For this review, take the finished solid that the model builds, in its own axes (mm). A direction names the side the tool comes from. Give positions to 0.01 mm unless a question says otherwise; leave off trailing zeros. Order: outer loops, then holes, each group sorted by start corner. A loop starts at its lowest first (then second) coordinate and runs counter-clockwise, first axis right, second up.
from build123d import *

# Parameters (mm, degrees)
SKETCH1_R           = 6.35
SKETCH1_R_2         = 7.62
BOSS_EXTRUDE1_DEPTH = 25.4
FILLET3_R           = 12.7


with BuildPart() as part:
    # Sketch1 → Boss-Extrude1 (new body)
    with BuildSketch(Plane.XY):
        Polygon((-106.967651581, 12.7), (103.301477372, 19.05), (125.298522628, 19.05), (136.297045256, 0), (125.298522628, -19.05), (103.301477372, -19.05), (-106.967651581, -12.7), (-121.632348419, -12.7), (-128.964696837, 0), (-121.632348419, 12.7), align=None)
        with Locations((-114.3, 0)):
            Circle(SKETCH1_R, mode=Mode.SUBTRACT)
        with Locations((114.3, 0)):
            Circle(SKETCH1_R_2, mode=Mode.SUBTRACT)
    extrude(amount=BOSS_EXTRUDE1_DEPTH)

    # Fillet3
    fillet3_edges = [part.edges().sort_by_distance(p)[0] for p in [
        (-128.964696837, 0, 12.7),
        (-121.632348419, 12.7, 12.7),
        (125.298522628, -19.05, 12.7),
        (136.297045256, 0, 12.7),
        (125.298522628, 19.05, 12.7),
        (-121.632348419, -12.7, 12.7),
    ]]
    fillet(fillet3_edges, radius=FILLET3_R - 0.0001)  # a hair under: the kernel refuses the full size


solid = part.part
1) To check wall thickness, follow line 1 (Y direction, x = 114.3, z = 13); line 2 (X direction, y = 1, z = 4.5); line 3 (Y direction, x = -114.3, z = 17.75). State the ranges of each line that lie inside material, in increasing order.
Answer sheet:
line 1: y = -19.05 to -7.62, 7.62 to 19.05
line 2: x = -126.96 to -120.57, -108.03 to 106.75, 121.85 to 134.29
line 3: y = -12.7 to -6.35, 6.35 to 12.7
2) Draft analysis for pull direction Y (two halves, no side actions). For faces 1 (the face through (124.4, -17.3, 12.9)), 2 (the face through (106.687, 0.335, 12.522)), 3 (the face through (134.332, 0.093, 12.878)), state which applies: +Y half, -Y half, draft (parallel to the pull), parting line (faces both ways), or undercut.
Answer sheet:
face 1: -Y half
face 2: undercut
face 3: parting line
3) Tool access review of faces 4 (the face through (-127, 0, 13)), 5 (the face through (-111, 12.7, 13)), 6 (the face through (-111, -12.7, 13)): name each direction out of +Z, -Z, +X, -X, +Y, -Y from which nothing blocks a thin tool from reaching the whole face with its end or side.
Answer sheet:
face 4: +Z, -Z, -X
face 5: +Z, -Z, -X, +Y
face 6: +Z, -Z, -X, -Y
4) We need section D-D on x = -34.5. Give the boundary of the cut face in (y, z), then the cut area to 3 significant figures.
Answer sheet:
outline: (-14.89, 0) - (14.89, 0) - (14.89, 25.4) - (-14.89, 25.4) - close
area: 756 mm2
5) We need section B-B on y = 0. Give the boundary of the cut face in (x, z), then the cut area to 3 significant figures.
Answer sheet:
outline: (-127, 0) - (-120.65, 0) - (-120.65, 25.4) - (-127, 25.4) - close; (-107.95, 0) - (106.68, 0) - (106.68, 25.4) - (-107.95, 25.4) - close; (121.92, 0) - (134.33, 0) - (134.33, 25.4) - (121.92, 25.4) - close
area: 5,930 mm2
6) We need section C-C on z = 21.25. Count the separate pieces of the cut face and the enclosed holes in it, then the cut area to 3 significant figures.
Answer sheet:
separate pieces: 1
enclosed holes: 2
area: 7,830 mm2
7) Clearance check with flat-ended pins moving along their axes: pin 1 (10 mm diameter, centred on y = -7.5, z = 8, fed in from -X); pin 2 (3.5 mm diameter, centred on x = -111, z = 17, fed in from +Y); pin 3 (8 mm diameter, centred on x = -41.5, z = 21, fed in from +Y). State where each tip first meets the part, or that it passes through.
Answer sheet:
pin 1: stops at x = -126.75
pin 2: stops at y = 12.7
pin 3: stops at y = 14.8
8) We need section A-A on x = 114.3. Give the boundary of the cut face in (y, z), then the cut area to 3 significant figures.
Answer sheet:
outline: (-19.05, 0) - (-7.62, 0) - (-7.62, 25.4) - (-19.05, 25.4) - close; (7.62, 0) - (19.05, 0) - (19.05, 25.4) - (7.62, 25.4) - close
area: 581 mm2
